```python
from build123d import *

# Parameters (mm, degrees)
SKETCH1_W           = 20
SKETCH1_H           = 32
BOSS_EXTRUDE1_DEPTH = 1
SKETCH2_R           = 10
BOSS_EXTRUDE2_DEPTH = 5
SKETCH3_R           = 1.5
CUT_EXTRUDE1_DEPTH  = 5
SKETCH4_R           = 7.5
BOSS_EXTRUDE3_DEPTH = 10
BOSS_EXTRUDE3_TAPER = 8
FILLET1_R           = 2


with BuildPart() as part:
    # Sketch1 → Boss-Extrude1 (new body)
    with BuildSketch(Plane(origin=(0, 0, 0), x_dir=(1, 0, 0), z_dir=(0, 1, 0))):
        Rectangle(SKETCH1_W, SKETCH1_H)
    extrude(amount=BOSS_EXTRUDE1_DEPTH)

    # Sketch2 → Boss-Extrude2 (add)
    with BuildSketch(Plane(origin=(0, 1, 0), x_dir=(1, 0, 0), z_dir=(0, 1, 0))):
        with Locations(Location((0, 4, 0), (0, 0, 180))):
            Circle(SKETCH2_R)
    extrude(amount=BOSS_EXTRUDE2_DEPTH)

    # Sketch3 → Cut-Extrude1 (cut)
    with BuildSketch(Plane(origin=(0, 1, 0), x_dir=(1, 0, 0), z_dir=(0, 1, 0))):
        with Locations(Location((8, 14, 0), (0, 0, 270))):
            Circle(SKETCH3_R)
        with Locations(Location((-8, 14, 0), (0, 0, 270))):
            Circle(SKETCH3_R)
        with Locations(Location((8, -14, 0), (0, 0, 270))):
            Circle(SKETCH3_R)
        with Locations(Location((-8, -14, 0), (0, 0, 270))):
            Circle(SKETCH3_R)
    extrude(amount=-CUT_EXTRUDE1_DEPTH, mode=Mode.SUBTRACT)

    # Sketch4 → Boss-Extrude3 (add)
    with BuildSketch(Plane(origin=(0, 6, 0), x_dir=(1, 0, 0), z_dir=(0, 1, 0))):
        with Locations((0, 4)):
            Circle(SKETCH4_R)
    extrude(amount=BOSS_EXTRUDE3_DEPTH, taper=BOSS_EXTRUDE3_TAPER)

    # Fillet1
    fillet1_edges = [part.edges().sort_by_distance(p)[0] for p in [
        (-6.094591653, 16, -4),
    ]]
    fillet(fillet1_edges, radius=FILLET1_R)


solid = part.part
```
The model under review builds one solid part; all positions refer to its coordinate system, in mm. A direction names the side the tool comes from. Round coordinates to 2 decimals unless told otherwise and drop trailing zeros. Write each loop counter-clockwise with the first axis right and the second up, starting at its lowest first coordinate (ties: lowest second). Pieces come first, ordered by that corner, then holes. Notation, with made-up numbers: (-28, 16.5) - (26, 16.5) arc R16 cw to (26, 37.5) - close; hole circle Ø7 at (15.25, 55). An arc over 180 degrees is marked (long way). Use one line per item in the form item = value.
Q1. Consider section B-B (x = 0). State the section outline as (y, z) points.
Answer key:
outline = (0, -16) - (1, -16) - (1, -14) - (6, -14) - (6, -11.5) - (14.28, -10.34) arc R2 ccw to (16, -8.36) - (16, 0.36) arc R2 ccw to (14.28, 2.34) - (6, 3.5) - (6, 6) - (1, 6) - (1, 16) - (0, 16) - close
Q2. Insertion check: pin 1 Ø6 at (x, y) = (8, 6) entering from -Z; pin 2 Ø2.5 at (x, z) = (-8, -14) entering from +Y; pin 3 Ø5 at (x, z) = (8, 14) entering from +Y; pin 4 Ø6 at (x, z) = (-8, -6.5) entering from +Y. Each pin has a flat end and moves straight along its axis. Give the tip position at first contact, or say it passes through.
Answer key:
pin_1 = -12.66
pin_2 = through
pin_3 = 1
pin_4 = 15.72
Q3. Consider section C-C (y = 2). State the section outline as (x, z) points.
Answer key:
outline = circle Ø20 at (0, -4)
Q4. For line 1 (X direction, y = 0.5, z = -14); line 2 (Y direction, x = 4.25, z = 9.5); line 3 (Y direction, x = 9.25, z = -6), list the stretches that pass through material, from the lowest coordinate up. Write a range as [from, to].
Answer key:
line_1 = [-10, -9.5], [-6.5, 6.5], [9.5, 10]
line_2 = [0, 1]
line_3 = [0, 6]
Q5. Tool access review of faces 4 (the flat face through (-4, 6, 3)), 5 (the flat face through (0, 1, 8)), 6 (the flat face through (-0.1, 0.5, -16)): name each direction out of +Z, -Z, +X, -X, +Y, -Y from which nothing blocks a thin tool from reaching the whole face with its end or side.
Answer key:
face_4 = +Y
face_5 = +Z, +Y
face_6 = -Z, +X, -X, +Y, -Y
Q6. Draft analysis for pull direction X (two halves, no side actions). For faces 1 (the flat face through (0, 1, -14.5)), 2 (the flat face through (-10, 0.5, 0.2)), 3 (the cylindrical face through (-8.9, 0.5, -15.2)), state which applies: +X half, -X half, draft (parallel to the pull), parting line (faces both ways), or undercut.
Answer key:
face_1 = draft
face_2 = -X half
face_3 = undercut
Q7. Consider section A-A (x = -8). State the section outline as (y, z) points, and give its area (3 significant figures).
Answer key:
outline = (0, -16) - (1, -16) - (1, -15.5) - (0, -15.5) - close; (0, -12.5) - (1, -12.5) - (1, -10) - (6, -10) - (6, 2) - (1, 2) - (1, 12.5) - (0, 12.5) - close; (0, 15.5) - (1, 15.5) - (1, 16) - (0, 16) - close
area = 86.0 mm2
Q8. Consider section D-D (z = 8). State the section outline as (x, y) points, and give its area (3 significant figures).
Answer key:
outline = (-10, 0) - (10, 0) - (10, 1) - (-10, 1) - close
area = 20.0 mm2
